from build123d import *

# Parameters (mm, degrees)
BOSS_EXTRUDE5_DEPTH = 400
SKETCH8_R           = 4.25
CUT_EXTRUDE1_DEPTH  = 9
SKETCH9_R           = 3
CUT_EXTRUDE2_DEPTH  = 12.3
LPATTERN1_COUNT     = 20
LPATTERN1_PITCH     = 60


with BuildPart() as part:
    # Sketch7 → Boss-Extrude5 (new body)
    with BuildSketch(Plane(origin=(58.5, 0, 0), x_dir=(0, 0, -1), z_dir=(1, 0, 0))):
        with BuildLine():
            Line((-7.709038211, 8.883084864), (-8.5, 8.601077183))
            Line((-8.5, 8.601077183), (-8.5, 6.104700538))
            ThreePointArc((-8.5, 6.104700538), (-8.566987298, 5.854700538), (-8.75, 5.671687836))
            Line((-8.75, 5.671687836), (-10, 4.95))
            Line((-10, 4.95), (-10, 1))
            Line((-10, 1), (-9, 0))
            Line((-9, 0), (-4, 0))
            Line((-4, 0), (-3.5, 0.5))
            Line((-3.5, 0.5), (3.5, 0.5))
            Line((3.5, 0.5), (4, 0))
            Line((4, 0), (9, 0))
            Line((9, 0), (10, 1))
            Line((10, 1), (10, 4.95))
            Line((10, 4.95), (8.75, 5.671687836))
            ThreePointArc((8.75, 5.671687836), (8.566987298, 5.854700538), (8.5, 6.104700538))
            Line((8.5, 6.104700538), (8.5, 8.46691323))
            Line((8.5, 8.46691323), (8.084678947, 8.882234283))
            ThreePointArc((8.084678947, 8.882234283), (6.941822875, 9.249266637), (6.503340774, 10.366659226))
            Line((6.503340774, 10.366659226), (6, 10.87))
            Line((6, 10.87), (6, 14.93))
            Line((6, 14.93), (6.503340774, 15.433340774))
            ThreePointArc((6.503340774, 15.433340774), (6.813545517, 16.412959034), (7.709038211, 16.916915136))
            Line((7.709038211, 16.916915136), (8.5, 17.198922817))
            Line((8.5, 17.198922817), (8.5, 19.3))
            Line((8.5, 19.3), (7.5, 20.3))
            Line((7.5, 20.3), (-7.5, 20.3))
            Line((-7.5, 20.3), (-8.5, 19.3))
            Line((-8.5, 19.3), (-8.5, 17.33308677))
            Line((-8.5, 17.33308677), (-8.084678947, 16.917765717))
            ThreePointArc((-8.084678947, 16.917765717), (-6.941822875, 16.550733363), (-6.503340774, 15.433340774))
            Line((-6.503340774, 15.433340774), (-6, 14.93))
            Line((-6, 14.93), (-6, 10.87))
            Line((-6, 10.87), (-6.503340774, 10.366659226))
            ThreePointArc((-6.503340774, 10.366659226), (-6.813545517, 9.387040966), (-7.709038211, 8.883084864))
        make_face()
    extrude(amount=BOSS_EXTRUDE5_DEPTH)

    # Sketch8 → Cut-Extrude1 (cut)
    with BuildSketch(Plane(origin=(0, 20.3, 0), x_dir=(1, 0, 0), z_dir=(0, 1, 0))):
        with Locations((79.1, 0)):
            Circle(SKETCH8_R)
    cut_extrude1 = extrude(amount=-CUT_EXTRUDE1_DEPTH, mode=Mode.SUBTRACT)

    # Sketch9 → Cut-Extrude2 (cut, through all)
    with BuildSketch(Plane(origin=(0, 11.3, 0), x_dir=(1, 0, 0), z_dir=(0, 1, 0))):
        with Locations((79.1, 0)):
            Circle(SKETCH9_R)
    cut_extrude2 = extrude(amount=-CUT_EXTRUDE2_DEPTH, mode=Mode.SUBTRACT)

    # LPattern1: Cut-Extrude1, Cut-Extrude2 ×20
    with Locations(*[(i * LPATTERN1_PITCH, 0, 0) for i in range(1, LPATTERN1_COUNT)]):
        add(cut_extrude1, mode=Mode.SUBTRACT)
        add(cut_extrude2, mode=Mode.SUBTRACT)


solid = part.part
Read the model definition and answer for the solid it produces. Units are mm, in the model's axes. A direction names the side the tool comes from. Give positions to 0.01 mm unless a question says otherwise; leave off trailing zeros. One line per item, written item: value. Start each with the question number.
(1) Flat-ended cylindrical pins translate along their axes: pin 1 Ø8 at (x, z) = (439.1, 0) entering from +Y; pin 2 Ø5 at (x, z) = (79.1, 0) entering from +Y; pin 3 Ø3 at (x, y) = (313, 12.5) entering from -Z; pin 4 Ø1.2 at (x, y) = (261.5, 14) entering from +Z. Find the tip coordinate at first contact, or state that the pin passes through.
(2) A tool of negligible diameter and unlimited length cuts with its end or side. For faces 1 (the flat face through (255.7, 0.5, 0)), 2 (the flat face through (316, 11.3, 1)), 3 (the flat face through (458.5, 10, 0)), from which of +Z, -Z, +X, -X, +Y, -Y can it reach the whole face along a straight path? Write none if from no direction.
(3) Find section A-A (z = 0). Give the number of separate pieces and of enclosed holes in the cut face, plus the area to 3 significant figures.
(4) Find the intervals of material crossed by line 1 (Z direction, x = 319.1, y = 2.5); line 2 (Y direction, x = 158.5, z = 7.5); line 3 (Y direction, x = 211, z = 3), in increasing order.
(5) Determine the mould class of faces 4 (the flat face through (58.5, 10, 0)), 5 (the flat face through (436, 11.3, 1)) for opening direction Z: pulls with the +Z half, pulls with the -Z half, needs draft (parallel to the pull), parting line crosses it, or undercut.
Results below:
1. pin 1: stops at y = 11.3
1. pin 2: passes through
1. pin 3: stops at z = -6
1. pin 4: stops at z = 6
2. face 1: +X, -X, -Y
2. face 2: +Y
2. face 3: +Z, -Z, +X, +Y, -Y
3. separate pieces: 8
3. enclosed holes: 0
3. area: 6,930 mm^2
4. line 1: z = -10 to -3, 3 to 10
4. line 2: y = 0 to 8.93, 16.87 to 20.3
4. line 3: y = 0.5 to 20.3
5. face 4: needs draft
5. face 5: undercut
